Source: CAD feature listing. Evaluate the final solid. Frame: model axes, mm. Round coordinates to 2 decimals unless told otherwise and drop trailing zeros. Order: outer loops, then holes, each group sorted by start corner. A loop starts at its lowest first (then second) coordinate and runs counter-clockwise, first axis right, second up. Notation, with made-up numbers: (-33.5, -26) -> (9.5, -26) arc R14 ccw to (9.5, -22) -> close; hole circle Ø5 at (-2, -15.5). An arc over 180 degrees is marked (long way). Write item = value, one per line. Start each with the question number.
(1) Ray query, line 1 (Z direction, x = 0, y = 1.75); line 2 (Z direction, x = 36, y = -1.25); line 3 (Z direction, x = 6, y = -1.25). Return the intervals inside material, ascending.
(2) Cut plane C-C on z = -42. Return the cut outline in (x, y) (3 decimals), then the cut area to 3 significant figures.
(3) Contact query for flat-ended pins moving along their axis: pin 1 Ø3 at (x, y) = (-4.5, -1.5) entering from -Z; pin 2 Ø2.5 at (x, z) = (-30, -30) entering from -Y; pin 3 Ø2 at (x, y) = (-19.5, 2.5) entering from +Z; pin 4 Ø1 at (x, y) = (-29, 2.5) entering from +Z. Output: stop coordinate, or through.
(4) Cut plane A-A on z = -18. Return the cut outline in (x, y) (3 decimals).
(5) Cut plane D-D on y = 1. Give the number of separate pieces and of enclosed holes in the cut face, then the cut area to 3 significant figures.
(6) Cut plane B-B on x = -18. Return the cut outline in (y, z) (3 decimals), then the cut area to 3 significant figures.
Autodesk Inventor part; units mm, degrees
ref_plane "YZ Plane" through (0, 0, 0) normal (1, 0, 0) x (0, 1, 0)
ref_plane "XZ Plane" through (0, 0, 0) normal (0, 1, 0) x (-1, 0, 0)
ref_plane "XY Plane" through (0, 0, 0) normal (0, 0, 1) x (1, 0, 0)
sketch "Sketch1" plane through (0, 0, 0) normal (0, 1, 0) x (-1, 0, 0)
  circle A0 centre (0, 0) radius 59.5
  dimension "d0" = 119
extrude "Extrusion1" add sketch "Sketch1" along normal mid plane 6.35
sketch "Sketch5" plane through (0, 3.175, 0) normal (0, 1, 0) x (1, 0, 0)
  circle A0 centre (-42, 0) radius 5
  circle A1 centre (-36, 6) radius 2
  circle A2 centre (-48, 6) radius 2
  circle A3 centre (-48, -6) radius 2
  circle A4 centre (-36, -6) radius 2
  circle A5 centre (0, -42) radius 5
  circle A6 centre (-6, -36) radius 2
  circle A7 centre (-6, -48) radius 2
  circle A8 centre (6, -48) radius 2
  circle A9 centre (6, -36) radius 2
  circle A10 centre (42, 0) radius 5
  circle A11 centre (36, -6) radius 2
  circle A12 centre (48, -6) radius 2
  circle A13 centre (48, 6) radius 2
  circle A14 centre (36, 6) radius 2
  circle A15 centre (0, 42) radius 5
  circle A16 centre (6, 36) radius 2
  circle A17 centre (6, 48) radius 2
  circle A18 centre (-6, 48) radius 2
  circle A19 centre (-6, 36) radius 2
  point P0 (0, 0)
  dimension "d37" = 10
  dimension "d38" = 42
  dimension "d39" = 4
  dimension "d40" = 6
  dimension "d41" = 6
  dimension "d44" = 360
  dimension "d48" = 360
extrude "Extrusion4" cut sketch "Sketch5" against normal through all
sketch "Sketch8" plane through (0, 3.175, 0) normal (0, 1, 0) x (1, 0, 0)
  circle A0 centre (-24, -24) radius 2.5
  circle A1 centre (-30, -18) radius 2
  circle A2 centre (-30, -30) radius 2
  circle A3 centre (-18, -30) radius 2
  circle A4 centre (-18, -18) radius 2
  circle A5 centre (24, -24) radius 2.5
  circle A6 centre (18, -30) radius 2
  circle A7 centre (30, -30) radius 2
  circle A8 centre (30, -18) radius 2
  circle A9 centre (18, -18) radius 2
  circle A10 centre (24, 24) radius 2.5
  circle A11 centre (30, 18) radius 2
  circle A12 centre (30, 30) radius 2
  circle A13 centre (18, 30) radius 2
  circle A14 centre (18, 18) radius 2
  circle A15 centre (-24, 24) radius 2.5
  circle A16 centre (-18, 30) radius 2
  circle A17 centre (-30, 30) radius 2
  circle A18 centre (-30, 18) radius 2
  circle A19 centre (-18, 18) radius 2
  circle A20 centre (-24, -24) radius 16
  circle A21 centre (24, -24) radius 16
  circle A22 centre (24, 24) radius 16
  circle A23 centre (-24, 24) radius 16
  point P0 (0, 0)
  dimension "d70" = 5
  dimension "d71" = 24
  dimension "d72" = 24
  dimension "d73" = 4
  dimension "d74" = 6
  dimension "d75" = 6
  dimension "d78" = 360
  dimension "d88" = 360
  dimension "d90" = 32
  dimension "d93" = 360
extrude "Extrusion6" cut sketch "Sketch8" against normal through all contours A0 | A1 | A2 | A3 | A4 | A5 | A6 | A7 | A8 | A9 | A10 | A11 | A12 | A13 | A14 | A15 | A16 | A17 | A18 | A19
properties part number "TurnTable"
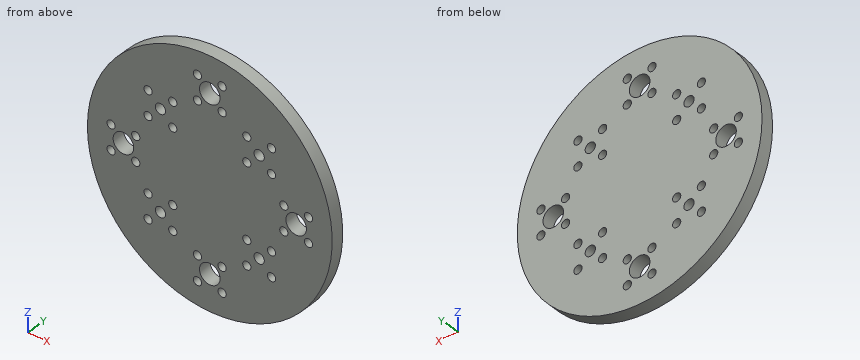
Evaluation:
q1.line_1 = -59.5 to -47, -37 to 37, 47 to 59.5
q1.line_2 = -47.37 to -8, -4 to 4, 8 to 47.37
q1.line_3 = -59.2 to -50, -46 to -38, -34 to 34, 38 to 46, 50 to 59.2
q2.outline = (-42.146, -3.175) -> (-5, -3.175) -> (-5, 3.175) -> (-42.146, 3.175) -> close; (5, -3.175) -> (42.146, -3.175) -> (42.146, 3.175) -> (5, 3.175) -> close
q2.area = 472 mm^2
q3.pin_1 = -59.42
q3.pin_2 = through
q3.pin_3 = 56.55
q3.pin_4 = 52.23
q4.outline = (-56.712, -3.175) -> (-32, -3.175) -> (-32, 3.175) -> (-56.712, 3.175) -> close; (-28, -3.175) -> (-20, -3.175) -> (-20, 3.175) -> (-28, 3.175) -> close; (-16, -3.175) -> (16, -3.175) -> (16, 3.175) -> (-16, 3.175) -> close; (20, -3.175) -> (28, -3.175) -> (28, 3.175) -> (20, 3.175) -> close; (32, -3.175) -> (56.712, -3.175) -> (56.712, 3.175) -> (32, 3.175) -> close
q5.separate_pieces = 1
q5.enclosed_holes = 40
q5.area = 10,300 mm^2
q6.outline = (-3.175, -56.712) -> (3.175, -56.712) -> (3.175, -32) -> (-3.175, -32) -> close; (-3.175, -28) -> (3.175, -28) -> (3.175, -20) -> (-3.175, -20) -> close; (-3.175, -16) -> (3.175, -16) -> (3.175, 16) -> (-3.175, 16) -> close; (-3.175, 20) -> (3.175, 20) -> (3.175, 28) -> (-3.175, 28) -> close; (-3.175, 32) -> (3.175, 32) -> (3.175, 56.712) -> (-3.175, 56.712) -> close
q6.area = 619 mm^2
